Build history of the part. All positions in model axes, mm. Face numbers are marked on the shaded views. A direction names the side the tool comes from. Give positions to 0.01 mm unless a question says otherwise; leave off trailing zeros. Order: outer loops, then holes, each group sorted by start corner. A loop starts at its lowest first (then second) coordinate and runs counter-clockwise, first axis right, second up. Notation, with made-up numbers: (19.5, 45) - (65.5, 45) arc R15 ccw to (65.5, 56) - close; hole circle Ø7 at (22.5, -5). An arc over 180 degrees is marked (long way). Answer in a Markdown table with one row per item.
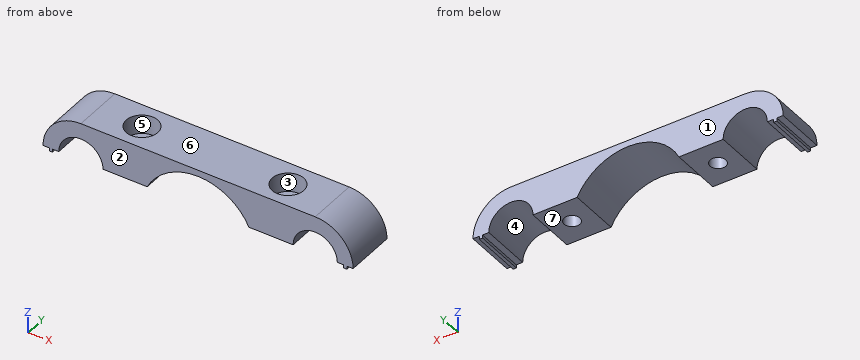
```python
from build123d import *

# Parameters (mm, degrees)
F1_DEPTH       = 8
F3_D           = 5
F3_CBORE_D     = 10
F3_CBORE_DEPTH = 6
F4_R           = 11.99999
F5_W           = 1
F5_H           = 16
F6_DEPTH       = 1
F7_W           = 1
F7_H           = 16
F8_DEPTH       = 1


# Not quite as in the source:
# - a fillet or chamfer is up to 0.001 mm smaller than in the source, because OpenCascade refuses the exact size
# - a feature names something its author has since deleted; it is built from what else it names


with BuildPart() as f1:
    # F0 (on Front) → F1 (new body, symmetric)
    with BuildSketch(Plane.XZ):
        with BuildLine():
            Line((-49.125, -6), (-44.125, -6))
            ThreePointArc((-44.125, -6), (-37.125, 1), (-30.125, -6))
            Line((-30.125, -6), (-16.1245154966, -6))
            ThreePointArc((-16.1245154966, -6), (0, 4), (16.1245154966, -6))
            Line((16.1245154966, -6), (30.125, -6))
            ThreePointArc((30.125, -6), (37.125, 1), (44.125, -6))
            Line((44.125, -6), (49.125, -6))
            Line((49.125, -6), (49.125, 6))
            Line((49.125, 6), (-49.125, 6))
            Line((-49.125, 6), (-49.125, -6))
        make_face()
    extrude(amount=F1_DEPTH, both=True)

    # F3 (through all)
    with Locations(Plane.XY.offset(6)):
        with Locations((-23.125, 0), (23.125, 0)):
            CounterBoreHole(F3_D / 2, F3_CBORE_D / 2, F3_CBORE_DEPTH)

    # F4 (radius 12 in the source; OpenCascade refuses exactly that, so slightly less here)
    f4_edges = [f1.edges().sort_by_distance(p)[0] for p in [
        (49.125, 0, 6),
        (-49.125, 0, 6),
    ]]
    fillet(f4_edges, radius=F4_R)

    # F5 (on face) → F6 (join)
    with BuildSketch(Plane(origin=(0, 0, -6), x_dir=(1, 0, 0), z_dir=(0, 0, -1))):
        with Locations((-46.625, 0)):
            Rectangle(F5_W, F5_H)
    extrude(amount=F6_DEPTH)

    # F7 (on face) → F8 (join)
    with BuildSketch(Plane(origin=(0, 0, -6), x_dir=(1, 0, 0), z_dir=(0, 0, -1))):
        with Locations((46.625, 0)):
            Rectangle(F7_W, F7_H)
    extrude(amount=F8_DEPTH)


solid = f1.part
```
1. Which spindle directions (+Z, -Z, +X, -X, +Y, -Y) get a long thin tool onto all of the face, cutting with end or side? Do the marked faces 5, 6 and 7. Say none if no direction does.
Check result:
| item | result |
|---|---|
| face 5 | +Z |
| face 6 | +Z, +X, -X, +Y, -Y |
| face 7 | -Z, +Y, -Y |
2. Cut at A-A on z = -3.25. Write the cut outline in (x, y) (3 decimals).
Check result:
| item | result |
|---|---|
| outline | (-48.806, -8) - (-43.562, -8) - (-43.562, 8) - (-48.806, 8) - close; (-30.688, -8) - (-14.437, -8) - (-14.437, 8) - (-30.688, 8) - close; (14.437, -8) - (30.688, -8) - (30.688, 8) - (14.437, 8) - close; (43.562, -8) - (48.806, -8) - (48.806, 8) - (43.562, 8) - close; hole circle Ø5 at (-23.125, 0); hole circle Ø5 at (23.125, 0) |
3. Cut at D-D on z = 5. Write the cut outline in (x, y) (3 decimals), and give its area (3 significant figures).
Check result:
| item | result |
|---|---|
| outline | (-41.921, -8) - (41.921, -8) - (41.921, 8) - (-41.921, 8) - close; hole circle Ø10 at (-23.125, 0); hole circle Ø10 at (23.125, 0) |
| area | 1,180 mm² |
4. Cut at C-C on y = 0. Count the separate pieces of the cut face and the enclosed holes in it, and give its area (3 significant figures).
Check result:
| item | result |
|---|---|
| separate pieces | 3 |
| enclosed holes | 0 |
| area | 555 mm² |
5. Two-plate mould, pull along Y, no slides. Class the marked faces 1, 2, 3 and 4: +Y half, -Y half, draft (parallel to the pull), parting line (faces both ways), or undercut.
Check result:
| item | result |
|---|---|
| face 1 | +Y half |
| face 2 | -Y half |
| face 3 | undercut |
| face 4 | draft |
6. Cut at B-B on x = -24. Write the cut outline in (y, z), and give its area (3 significant figures).
Check result:
| item | result |
|---|---|
| outline | (-8, -6) - (-2.34, -6) - (-2.34, 0) - (-4.92, 0) - (-4.92, 6) - (-8, 6) - close; (2.34, -6) - (8, -6) - (8, 6) - (4.92, 6) - (4.92, 0) - (2.34, 0) - close |
| area | 105 mm² |
7. Drop flat-ended pins along their axis: P1, Ø5, axis at y = -0.5, z = 0.5, coming from the +X side; P2, Ø4.5, axis at x = -23.125, y = 0, coming from the +Z side; P3, Ø9, axis at x = 23.125, y = 0, coming from the -Z side; P4, Ø6.5, axis at x = 23.125, y = 0, coming from the +Z side. Give the stop position or say it passes through.
Check result:
| item | result |
|---|---|
| P1 | stops at x = 48.44 |
| P2 | passes through |
| P3 | stops at z = -6 |
| P4 | stops at z = 0 |
8. Probe line 1 (X direction, y = 4.5, z = -1.5); line 2 (Y direction, x = -23, z = -3.5); line 3 (Z direction, x = 18.5, y = 7). List the from-to ranges inside material, lowest first.
Check result:
| item | result |
|---|---|
| line 1 | x = -48.25 to -42.49, -31.76 to -12.95, 12.95 to 31.76, 42.49 to 48.25 |
| line 2 | y = -8 to -2.5, 2.5 to 8 |
| line 3 | z = -6 to 6 |
